from build123d import *

# Parameters (mm, degrees)
SKETCH2_W            = 47
SKETCH2_H            = 25
BOSS_EXTRUDE1_DEPTH  = 11
BOSS_EXTRUDE2_DEPTH  = 25
SKETCH4_W            = 21
SKETCH4_H            = 11
CUT_EXTRUDE1_DEPTH   = 5
SKETCH5_R            = 2.5
SKETCH6_R            = 1.25
CHAMFER1_SIZE        = 1
SKETCH7_W            = 0.855148952
SKETCH7_H            = 0.908595762
BOSS_EXTRUDE3_DEPTH  = 5
LPATTERN1_COUNT      = 7
LPATTERN1_PITCH      = 2.833333333
LPATTERN1_COUNT_DIR2 = 3
LPATTERN1_PITCH_DIR2 = 3.5


with BuildPart() as part:
    # Sketch2 → Boss-Extrude1 (new body)
    with BuildSketch(Plane(origin=(0, 0, 0), x_dir=(1, 0, 0), z_dir=(0, 1, 0))):
        Rectangle(SKETCH2_W, SKETCH2_H)
    extrude(amount=BOSS_EXTRUDE1_DEPTH)

    # Sketch3 → Boss-Extrude2 (add)
    with BuildSketch(Plane.XY.offset(12.5)):
        Polygon((-23.5, 11), (-9.5, 11), (-12.5, 15), (-23.5, 15), align=None)
    extrude(amount=-BOSS_EXTRUDE2_DEPTH)

    # Sketch4 → Cut-Extrude1 (cut)
    with BuildSketch(Plane.ZY.offset(23.5)):
        with Locations((0, 7.5)):
            Rectangle(SKETCH4_W, SKETCH4_H)
    extrude(amount=-CUT_EXTRUDE1_DEPTH, mode=Mode.SUBTRACT)

    # Sketch5 → Loft1 section 0
    with BuildSketch(Plane(origin=(23.5, 0, 0), x_dir=(0, 0, -1), z_dir=(1, 0, 0))):
        with Locations((-7.5, 5.5)):
            Circle(SKETCH5_R)
    # Sketch6 → Loft1 section 1
    with BuildSketch(Plane(origin=(27.5, 0, 0), x_dir=(0, 0, -1), z_dir=(1, 0, 0))):
        with Locations((-7.5, 5.5)):
            Circle(SKETCH6_R)
    loft1 = loft()

    # Mirror1: Loft1 across plane
    add(loft1.mirror(Plane.XY))

    # Chamfer1
    chamfer1_edges = [part.edges().sort_by_distance(p)[0] for p in [
        (7, 11, 12.5),
        (-23.5, 15, 0),
        (-11, 13, 12.5),
        (-18, 15, 12.5),
        (-18, 15, -12.5),
        (-11, 13, -12.5),
        (23.5, 11, 0),
        (0, 0, 12.5),
        (-23.5, 0, 0),
        (0, 0, -12.5),
        (23.5, 0, 0),
        (23.5, 5.5, 12.5),
        (-23.5, 7.5, 12.5),
        (-23.5, 7.5, -12.5),
        (23.5, 5.5, -12.5),
        (7, 11, -12.5),
    ]]
    chamfer(chamfer1_edges, length=CHAMFER1_SIZE)

    # Sketch7 → Boss-Extrude3 (add)
    with BuildSketch(Plane.ZY.offset(18.5)):
        with Locations((-8.5, 4)):
            Rectangle(SKETCH7_W, SKETCH7_H)
    boss_extrude3 = extrude(amount=BOSS_EXTRUDE3_DEPTH)

    # LPattern1: Boss-Extrude3 7 × 3
    with Locations(*[(0, j * LPATTERN1_PITCH_DIR2, i * LPATTERN1_PITCH) for i in range(LPATTERN1_COUNT) for j in range(LPATTERN1_COUNT_DIR2) if (i, j) != (0, 0)]):
        add(boss_extrude3)


solid = part.part
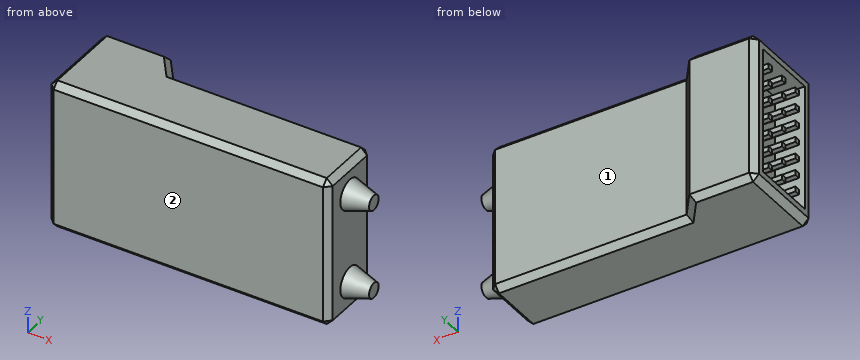
Build history of the part. All positions in model axes, mm. Face numbers are marked on the shaded views. A direction names the side the tool comes from. Round coordinates to 2 decimals unless told otherwise and drop trailing zeros. Write each loop counter-clockwise with the first axis right and the second up, starting at its lowest first coordinate (ties: lowest second). Pieces come first, ordered by that corner, then holes. Notation, with made-up numbers: (69, 56) -> (97, 56) arc R29 cw to (97, 92) -> close; hole circle Ø6 at (65, 25.25). An arc over 180 degrees is marked (long way). Write item = value, one per line.
(1) Band-saw the part on C-C (y = 8.5). Give the cut face in (x, z).
Answer:
outline = (-23.5, -11.5) -> (-22.5, -12.5) -> (22.5, -12.5) -> (23.5, -11.5) -> (23.5, 11.5) -> (22.5, 12.5) -> (-22.5, 12.5) -> (-23.5, 11.5) -> (-23.5, 10.5) -> (-18.5, 10.5) -> (-18.5, -10.5) -> (-23.5, -10.5) -> close
(2) Band-saw the part on B-B (x = 14). Give the cut face in (y, z).
Answer:
outline = (0, -11.5) -> (1, -12.5) -> (10, -12.5) -> (11, -11.5) -> (11, 11.5) -> (10, 12.5) -> (1, 12.5) -> (0, 11.5) -> close
(3) Band-saw the part on A-A (z = -11). Give the cut face in (x, y).
Answer:
outline = (-23.5, 1) -> (-22.5, 0) -> (22.5, 0) -> (23.5, 1) -> (23.5, 10) -> (22.5, 11) -> (-9.5, 11) -> (-12.5, 15) -> (-22.5, 15) -> (-23.5, 14) -> close
(4) Tool access for the marked faces 1 and 2: list every direction of +Z, -Z, +X, -X, +Y, -Y with a clear straight run to the whole face (end or side of a thin tool).
Answer:
face_1 = +Z, -Z, +X, +Y
face_2 = +Z, -Z, +X, -X, -Y
(5) Flat gauge pins, fed straight in: pin 1 (6 mm diameter, centred on x = 20, z = -2, fed in from +Y); pin 2 (2 mm diameter, centred on y = 5.5, z = 7.5, fed in from -X). Where does each tip first touch, or does it go through?
Answer:
pin_1 = 11
pin_2 = -18.5
(6) Probe L1, parallel to Y at x = -20, z = 6.5; L2, parallel to Y at x = -9, z = 8.5; L3, parallel to X at y = 9.75, z = -9. List the from-to ranges inside material, lowest first.
Answer:
L1 = 0 to 2, 13 to 15
L2 = 0 to 11
L3 = -18.5 to 23.5
(7) Band-saw the part on D-D (z = 7.5). Give the cut face in (x, y).
Answer:
outline = (-23.5, 1) -> (-22.5, 0) -> (22.5, 0) -> (23.5, 1) -> (23.5, 3) -> (27.5, 4.25) -> (27.5, 6.75) -> (23.5, 8) -> (23.5, 10) -> (22.5, 11) -> (-9.5, 11) -> (-12.5, 15) -> (-22.5, 15) -> (-23.5, 14) -> (-23.5, 13) -> (-18.5, 13) -> (-18.5, 2) -> (-23.5, 2) -> close
